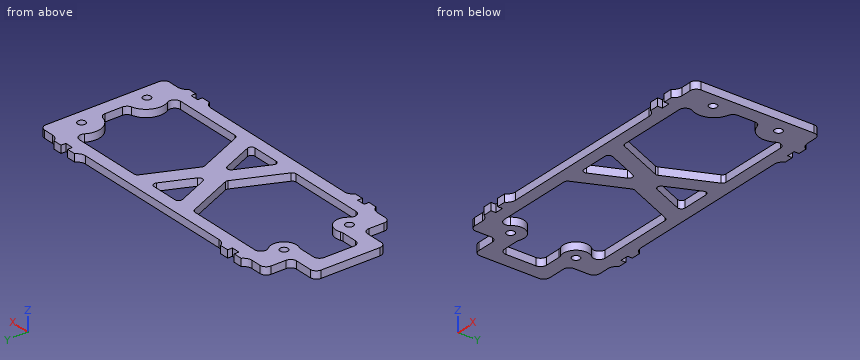
from build123d import *

# Parameters (mm, degrees)
SKETCH1_R           = 0.824992
BOSS_EXTRUDE1_DEPTH = 1.5875
FILLET4_R           = 0.762
FILLET5_R           = 1.27
FILLET6_R           = 1.905


with BuildPart() as part:
    # Sketch1 → Boss-Extrude1 (new body)
    with BuildSketch(Plane.XY):
        Polygon((-7.7520038, 24.7080024), (-12.8634998, 24.7080024), (-12.8634998, 25.7240024), (-14.7684998, 25.7240024), (-14.7684998, 24.7080024), (-16.5464998, 24.7080024), (-16.5464998, 25.7240024), (-18.4514998, 25.7240024), (-18.4514998, 24.7080024), (-38.1999998, 24.7080024), (-57.9484998, 24.7080024), (-57.9484998, 25.7240024), (-59.8534998, 25.7240024), (-59.8534998, 24.7080024), (-61.6314998, 24.7080024), (-61.6314998, 25.7240024), (-63.5364998, 25.7240024), (-63.5364998, 24.7080024), (-68.6479958, 24.7080024), (-68.6479958, 18.9868048), (-74.8538, 18.9868048), (-74.8538, 11.5000024), (-74.8538, 4.0132), (-68.6479958, 4.0132), (-68.6479958, -1.7079976), (-63.5364998, -1.7079976), (-63.5364998, -2.7239976), (-61.6314998, -2.7239976), (-61.6314998, -1.7079976), (-59.8534998, -1.7079976), (-59.8534998, -2.7239976), (-57.9484998, -2.7239976), (-57.9484998, -1.7079976), (-38.1999998, -1.7079976), (-18.4514998, -1.7079976), (-18.4514998, -2.7239976), (-16.5464998, -2.7239976), (-16.5464998, -1.7079976), (-14.7684998, -1.7079976), (-14.7684998, -2.7239976), (-12.8634998, -2.7239976), (-12.8634998, -1.7079976), (-7.7520038, -1.7079976), (-7.7520038, 11.5000024), align=None)
        with Locations((-10.8000038, 18.2999888)):
            Circle(SKETCH1_R, mode=Mode.SUBTRACT)
        with Locations((-10.8000038, 4.499991)):
            Circle(SKETCH1_R, mode=Mode.SUBTRACT)
        with Locations((-65.5999958, 18.2999888)):
            Circle(SKETCH1_R, mode=Mode.SUBTRACT)
        with Locations((-65.5999958, 4.499991)):
            Circle(SKETCH1_R, mode=Mode.SUBTRACT)
        with BuildLine():
            Line((-68.6479958, 15.9388048), (-71.8058, 15.9388048))
            Line((-71.8058, 15.9388048), (-71.8058, 11.5000024))
            Line((-71.8058, 11.5000024), (-71.8058, 7.0612))
            Line((-71.8058, 7.0612), (-68.6479958, 7.0612))
            Line((-68.6479958, 7.0612), (-67.121334605, 7.0612))
            ThreePointArc((-67.121334605, 7.0612), (-66.871048858, 7.086106813), (-66.630580151, 7.159850323))
            ThreePointArc((-66.630580151, 7.159850323), (-63.434712075, 6.257075855), (-63.596128623, 2.940071303))
            ThreePointArc((-63.596128623, 2.940071303), (-63.798895247, 1.578288502), (-62.641906157, 0.8320024))
            Line((-62.641906157, 0.8320024), (-45.934562137, 0.8320024))
            Line((-45.934562137, 0.8320024), (-41.2479998, 11.5000024))
            Line((-41.2479998, 11.5000024), (-45.934562137, 22.1680024))
            Line((-45.934562137, 22.1680024), (-62.641906157, 22.1680024))
            ThreePointArc((-62.641906157, 22.1680024), (-63.798895247, 21.421716298), (-63.596128623, 20.059933497))
            ThreePointArc((-63.596128623, 20.059933497), (-63.434712075, 16.742928945), (-66.630580151, 15.840154477))
            ThreePointArc((-66.630580151, 15.840154477), (-66.871048858, 15.913897987), (-67.121334605, 15.9388048))
            Line((-67.121334605, 15.9388048), (-68.6479958, 15.9388048))
        make_face(mode=Mode.SUBTRACT)
        with BuildLine():
            Line((-10.8000038, 13.316268632), (-10.8000038, 9.683736168))
            ThreePointArc((-10.8000038, 9.683736168), (-11.067211137, 8.904437204), (-11.756392579, 8.453066431))
            ThreePointArc((-11.756392579, 8.453066431), (-14.373483224, 6.193438859), (-14.142504388, 2.743550602))
            ThreePointArc((-14.142504388, 2.743550602), (-14.136809019, 1.470284986), (-15.238549964, 0.8320024))
            Line((-15.238549964, 0.8320024), (-30.465437463, 0.8320024))
            Line((-30.465437463, 0.8320024), (-35.1519998, 11.5000024))
            Line((-35.1519998, 11.5000024), (-30.465437463, 22.1680024))
            Line((-30.465437463, 22.1680024), (-15.238549964, 22.1680024))
            ThreePointArc((-15.238549964, 22.1680024), (-14.136809019, 21.529719814), (-14.142504388, 20.256454198))
            ThreePointArc((-14.142504388, 20.256454198), (-14.373483224, 16.806565941), (-11.756392579, 14.546938369))
            ThreePointArc((-11.756392579, 14.546938369), (-11.067211137, 14.095567596), (-10.8000038, 13.316268632))
        make_face(mode=Mode.SUBTRACT)
        Polygon((-42.217053232, 22.1680024), (-38.1999998, 13.0240024), (-34.182946368, 22.1680024), align=None, mode=Mode.SUBTRACT)
        Polygon((-34.182946368, 0.8320024), (-38.1999998, 9.9760024), (-42.217053232, 0.8320024), align=None, mode=Mode.SUBTRACT)
    extrude(amount=BOSS_EXTRUDE1_DEPTH)

    # Fillet4
    fillet4_edges = [part.edges().sort_by_distance(p)[0] for p in [
        (-34.182946368, 22.1680024, 0.79375),
        (-42.217053232, 22.1680024, 0.79375),
        (-38.1999998, 13.0240024, 0.79375),
        (-45.934562137, 0.8320024, 0.79375),
        (-41.2479998, 11.5000024, 0.79375),
        (-45.934562137, 22.1680024, 0.79375),
        (-30.465437463, 22.1680024, 0.79375),
        (-35.1519998, 11.5000024, 0.79375),
        (-30.465437463, 0.8320024, 0.79375),
        (-42.217053232, 0.8320024, 0.79375),
        (-34.182946368, 0.8320024, 0.79375),
        (-38.1999998, 9.9760024, 0.79375),
    ]]
    fillet(fillet4_edges, radius=FILLET4_R)

    # Fillet5
    fillet5_edges = [part.edges().sort_by_distance(p)[0] for p in [
        (-71.8058, 15.9388048, 0.79375),
        (-71.8058, 7.0612, 0.79375),
        (-7.7520038, -1.7079976, 0.79375),
        (-68.6479958, -1.7079976, 0.79375),
        (-68.6479958, 4.0132, 0.79375),
        (-74.8538, 4.0132, 0.79375),
        (-74.8538, 18.9868048, 0.79375),
        (-68.6479958, 18.9868048, 0.79375),
        (-68.6479958, 24.7080024, 0.79375),
        (-7.7520038, 24.7080024, 0.79375),
    ]]
    fillet(fillet5_edges, radius=FILLET5_R)

    # Fillet6
    # the kernel refuses this fillet: 1.905 mm, written as the material it adds along each edge
    with BuildSketch(Plane(origin=(-18.4514998, -1.7079976, 0), x_dir=(0, -1, 0), z_dir=(0, 0, 1)), Plane(origin=(-63.5364998, -1.7079976, 0), x_dir=(0, -1, 0), z_dir=(0, 0, 1))) as fillet6_piece_1:
        with BuildLine():
            CenterArc((1.905, -1.684845394), FILLET6_R, 117.818139285, 62.181860715)
            Line((0, -1.684845394), (-0.0381, -1.684845394))
            Line((-0.0381, -1.684845394), (-0.0381, 0))
            Line((-0.0381, 0), (0, 0.0381))
            ThreePointArc((0, 0.0381), (0.508, 0.0381), (0.99822, 0.033696908))
            Line((0.99822, 0.033696908), (1.016, 0))
        make_face()
    extrude(amount=1.5875)
    with BuildSketch(Plane(origin=(-12.8634998, -1.7079976, 0), x_dir=(1, 0, 0), z_dir=(0, 0, 1)), Plane(origin=(-57.9484998, -1.7079976, 0), x_dir=(1, 0, 0), z_dir=(0, 0, 1))) as fillet6_piece_2:
        with BuildLine():
            CenterArc((1.684845394, -1.905), FILLET6_R, 90, 62.181860715)
            Line((0, -1.016), (-0.033696908, -0.99822))
            ThreePointArc((-0.033696908, -0.99822), (-0.0381, -0.508), (-0.0381, 0))
            Line((-0.0381, 0), (0, 0.0381))
            Line((0, 0.0381), (1.684845394, 0.0381))
            Line((1.684845394, 0.0381), (1.684845394, 0))
        make_face()
    extrude(amount=1.5875)
    with BuildSketch(Plane(origin=(-18.4514998, 24.7080024, 0), x_dir=(0, 1, 0), z_dir=(0, 0, 1)), Plane(origin=(-63.5364998, 24.7080024, 0), x_dir=(0, 1, 0), z_dir=(0, 0, 1))) as fillet6_piece_3:
        with BuildLine():
            CenterArc((1.905, 1.684845394), FILLET6_R, 180, 62.181860715)
            Line((0, 1.684845394), (-0.0381, 1.684845394))
            Line((-0.0381, 1.684845394), (-0.0381, 0))
            Line((-0.0381, 0), (0, -0.0381))
            ThreePointArc((0, -0.0381), (0.508, -0.0381), (0.99822, -0.033696908))
            Line((0.99822, -0.033696908), (1.016, 0))
        make_face()
    extrude(amount=1.5875)
    with BuildSketch(Plane(origin=(-12.8634998, 24.7080024, 0), x_dir=(1, 0, 0), z_dir=(0, 0, 1)), Plane(origin=(-57.9484998, 24.7080024, 0), x_dir=(1, 0, 0), z_dir=(0, 0, 1))) as fillet6_piece_4:
        with BuildLine():
            CenterArc((1.684845394, 1.905), FILLET6_R, 207.818139285, 62.181860715)
            Line((0, 1.016), (-0.033696908, 0.99822))
            ThreePointArc((-0.033696908, 0.99822), (-0.0381, 0.508), (-0.0381, 0))
            Line((-0.0381, 0), (0, -0.0381))
            Line((0, -0.0381), (1.684845394, -0.0381))
            Line((1.684845394, -0.0381), (1.684845394, 0))
        make_face()
    extrude(amount=1.5875)


solid = part.part
Source: CAD feature listing. Evaluate the final solid. Frame: model axes, mm. Coordinates: 2 decimals unless noted, no trailing zeros. Loops run counter-clockwise (first coordinate to the right, second up) from the corner with the lowest first, then second, coordinate; pieces in that order, holes last. Notation, with made-up numbers: (-20, 56) -> (15, 56) arc R18 ccw to (15, 79) -> close; hole circle Ø6 at (89, -33.5). An arc over 180 degrees is marked (long way). Answer in a Markdown table with one row per item. Add a question column.
Q1. Section A-A on x = -26. Return the cut outline in (y, z).
Q2. Contact query for flat-ended pins moving along their axis: pin 1 Ø0.5 at (y, z) = (22.5, 0.5) entering from -X; pin 2 Ø0.5 at (x, z) = (-57, 1) entering from +Y; pin 3 Ø0.8 at (y, z) = (25.5, 1) entering from +X. Output: stop coordinate, or through.
Q3. Ray query, line 1 along Y through (x, z) = (-22, 0.5); line 2 along X through (y, z) = (19.5, 1.5); line 3 along Y through (x, z) = (-36.5, 1). Return the intervals inside material, ascending.
Q4. Section B-B on z = 1.3. Give the number of separate pieces and of enclosed holes in the cut face, and give its area (3 significant figures).
Computed values:
| question | item | result |
|---|---|---|
| 1 | outline | (-1.71, 0) -> (0.83, 0) -> (0.83, 1.59) -> (-1.71, 1.59) -> close; (22.17, 0) -> (24.71, 0) -> (24.71, 1.59) -> (22.17, 1.59) -> close |
| 2 | pin 1 | stops at x = -68.65 |
| 2 | pin 2 | stops at y = 24.98 |
| 2 | pin 3 | stops at x = -12.34 |
| 3 | line 1 | y = -1.71 to 0.83, 22.17 to 24.71 |
| 3 | line 2 | x = -68.9 to -63.22, -44.76 to -41.04, -35.36 to -31.64, -14.48 to -7.75 |
| 3 | line 3 | y = -1.71 to 0.83, 6.11 to 16.89, 22.17 to 24.71 |
| 4 | separate pieces | 1 |
| 4 | enclosed holes | 8 |
| 4 | area | 726 mm^2 |
